```python
from build123d import *

# Parameters (mm, degrees)
SKETCH1_W             = 990
SKETCH1_H             = 420
BOSS_EXTRUDE1_DEPTH   = 241.3
BOSS_EXTRUDE2_START   = 12.7
SKETCH2_R             = 139.7
BOSS_EXTRUDE2_DEPTH   = 114.3
BOSS_EXTRUDE2_2_DEPTH = 114.3
BOSS_EXTRUDE3_REACH   = 872.36
SKETCH3_R             = 25.4
CHAMFER1_SIZE         = 127


with BuildPart() as part:
    # Sketch1 → Boss-Extrude1 (new body)
    with BuildSketch(Plane(origin=(0, 0, 0), x_dir=(1, 0, 0), z_dir=(0, 1, 0))):
        Rectangle(SKETCH1_W, SKETCH1_H)
    extrude(amount=BOSS_EXTRUDE1_DEPTH)


with BuildPart() as body_2:
    # Sketch2 → Boss-Extrude2 (new body)
    with BuildSketch(Plane.XY.offset(210).offset(BOSS_EXTRUDE2_START)):
        with Locations((-355.3, 0)):
            Circle(SKETCH2_R)
    extrude(amount=BOSS_EXTRUDE2_DEPTH)


with BuildPart() as body_3:
    # Sketch2 → Boss-Extrude2 2 (new body)
    with BuildSketch(Plane.XY.offset(210).offset(BOSS_EXTRUDE2_START)):
        with Locations((355.3, 0)):
            Circle(SKETCH2_R)
    extrude(amount=BOSS_EXTRUDE2_2_DEPTH)


with BuildPart() as body_4:
    # Mirror2: mirrored copy
    add(body_3.part.mirror(Plane.XY))

    # Boss-Extrude3: up to this face of the body (flat: up to its plane)
    boss_extrude3_end = Plane(body_4.part.faces().sort_by_distance((355.3, 0, -337))[0])
    # Sketch3 → Boss-Extrude3 (add, up to the picked face)
    with BuildSketch(Plane.XY.offset(337), mode=Mode.PRIVATE) as boss_extrude3_sk1:
        with Locations((-355.3, 0)):
            Circle(SKETCH3_R)
    boss_extrude3_tool1 = split(extrude(boss_extrude3_sk1.sketch, amount=-BOSS_EXTRUDE3_REACH, mode=Mode.PRIVATE), bisect_by=boss_extrude3_end, keep=Keep.BOTH, mode=Mode.PRIVATE)
    # Sketch3 → Boss-Extrude3 (add, up to the picked face)
    with BuildSketch(Plane.XY.offset(337), mode=Mode.PRIVATE) as boss_extrude3_sk2:
        with Locations((355.3, 0)):
            Circle(SKETCH3_R)
    boss_extrude3_tool2 = split(extrude(boss_extrude3_sk2.sketch, amount=-BOSS_EXTRUDE3_REACH, mode=Mode.PRIVATE), bisect_by=boss_extrude3_end, keep=Keep.BOTH, mode=Mode.PRIVATE)

    add(part.part)  # Boss-Extrude3 merges part

    add(body_2.part)  # Boss-Extrude3 merges body 2

    add(body_3.part)  # Boss-Extrude3 merges body 3


with BuildPart() as body_5:
    # Mirror2 2: mirrored copy
    add(body_2.part.mirror(Plane.XY))


with BuildPart() as body_4_1:
    add(body_4.part)

    add(body_5.part)  # Boss-Extrude3 merges body 5
    add(boss_extrude3_tool1.solids().sort_by(Axis((-355.3, 0, 337), (0, 0, -1)))[0])
    add(boss_extrude3_tool2.solids().sort_by(Axis((355.3, 0, 337), (0, 0, -1)))[0])

    # Chamfer1
    chamfer1_edges = [body_4_1.edges().sort_by_distance(p)[0] for p in [
        (495, 241.3, 0),
    ]]
    chamfer(chamfer1_edges, length=CHAMFER1_SIZE)


solid = body_4_1.part
```
Build history of the part. All positions in model axes, mm. A direction names the side the tool comes from. Round coordinates to 2 decimals unless told otherwise and drop trailing zeros. Loops run counter-clockwise (first coordinate to the right, second up) from the corner with the lowest first, then second, coordinate; pieces in that order, holes last.
Item 1: Two-plate mould, pull along X, no slides. Class faces 6 (the face through (-222.05, 41.96, 279.05)), 7 (the face through (353, 2, 337)), 8 (the face through (495, 56, 3)), 9 (the face through (-5, 0, -3)): released by +X, released by -X, zero draft, split by the parting line, or undercut.
Item 2: Saw through at B-B (y = 70). List the corners of the cut face in (x, z).
Item 3: Pin check, flat tips, straight feed: P1, Ø12, axis at x = 130.5, z = -127.5, coming from the -Y side; P2, Ø4, axis at x = 33.5, y = 165.5, coming from the +Z side; P3, Ø12, axis at x = 220, y = 102.5, coming from the -Z side. Stop position of each tip, or through.
Item 4: Drill centre lines: line 1 along Z through (x, y) = (-304, -5); line 2 along Z through (x, y) = (-139, 169); line 3 along Y through (x, z) = (-40, 201). Where is each one in solid material? Low to high.
Item 5: Saw through at D-D (z = -99). List the corners of the cut face in (x, y), then the cut area to 3 significant figures.
Item 6: Which spindle directions (+Z, -Z, +X, -X, +Y, -Y) get a long thin tool onto all of the face, cutting with end or side? Do faces 1 (the face through (-357, 2, 337)), 2 (the face through (-439, 0, -3)), 3 (the face through (-222.05, 41.96, -279.05)), 4 (the face through (430.6, 178.7, 2.9)), 5 (the face through (437, 0, -3)). Say none if no direction does.
Item 7: Saw through at A-A (x = -248.5). List the corners of the cut face in (y, z), then the cut area to 3 significant figures.
Item 8: Saw through at C-C (x = 355.3). List the corners of the cut face in (y, z), then the cut area to 3 significant figures.
Worked answers:
1. face 6: undercut
1. face 7: zero draft
1. face 8: released by +X
1. face 9: undercut
2. outline: (-495, -210) - (495, -210) - (495, 210) - (-495, 210) - close; (-476.2, -337) - (-234.4, -337) - (-234.4, -222.7) - (-476.2, -222.7) - close; (-476.2, 222.7) - (-234.4, 222.7) - (-234.4, 337) - (-476.2, 337) - close; (234.4, -337) - (476.2, -337) - (476.2, -222.7) - (234.4, -222.7) - close; (234.4, 222.7) - (476.2, 222.7) - (476.2, 337) - (234.4, 337) - close
3. P1: stops at y = 0
3. P2: stops at z = 210
3. P3: stops at z = -210
4. line 1: z = -337 to -222.7, 222.7 to 337
4. line 2: z = -210 to 210
4. line 3: y = 0 to 241.3
5. outline: (-495, 0) - (-380.7, 0) arc R25.4 ccw to (-329.9, 0) - (329.9, 0) arc R25.4 ccw to (380.7, 0) - (495, 0) - (495, 114.3) - (368, 241.3) - (-495, 241.3) - close
5. area: 233,000 mm2
6. face 1: +Z, +X, -X, +Y, -Y
6. face 2: -X, -Y
6. face 3: -Z
6. face 4: +Z, -Z, +X, +Y
6. face 5: +X, -Y
7. outline: (-90.05, -337) - (90.05, -337) - (90.05, -222.7) - (-90.05, -222.7) - close; (-90.05, 222.7) - (90.05, 222.7) - (90.05, 337) - (-90.05, 337) - close; (0, -210) - (241.3, -210) - (241.3, 210) - (0, 210) - close
7. area: 143,000 mm2
8. outline: (-139.7, -337) - (139.7, -337) - (139.7, -222.7) - (25.4, -222.7) - (25.4, -210) - (241.3, -210) - (241.3, 210) - (25.4, 210) - (25.4, 222.7) - (139.7, 222.7) - (139.7, 337) - (-139.7, 337) - (-139.7, 222.7) - (-25.4, 222.7) - (-25.4, -222.7) - (-139.7, -222.7) - close
8. area: 177,000 mm2
